Drawing for the job (mm, zero at the part's lowest x, y, z). A direction names the side the tool comes from. Give positions to 0.01 mm unless a question says otherwise; leave off trailing zeros. Order: outer loops, then holes, each group sorted by start corner. A loop starts at its lowest first (then second) coordinate and runs counter-clockwise, first axis right, second up. Notation, with made-up numbers: (89.25, 46.25) - (143.25, 46.25) arc R12 cw to (143.25, 68.25) - close; hole circle Ø9 at (45, 19). An arc over 180 degrees is marked (long way). Use CSV: the item, a comma, the result in double quotes. Start each with the question number.
(1) Band-saw the part on B-B, the plane x = 3.66. Give the cut face in (y, z).
(2) Band-saw the part on D-D, the plane x = 23.66. Give the cut face in (y, z), then the cut area to 3 significant figures.
(3) Band-saw the part on A-A, the plane y = 17. Give the cut face in (x, z), then the cut area to 3 significant figures.
(4) Drop flat-ended pins along their axis: pin 1 Ø6 at (x, y) = (41.5, 30.5) entering from -Z; pin 2 Ø2.5 at (x, z) = (5, 3.5) entering from +Y; pin 3 Ø1.5 at (x, z) = (3, 2) entering from -Y; pin 4 Ø2 at (x, y) = (12.5, 20.5) entering from +Z. Give the stop position or say it passes through.
(5) Pull direction X, two halves, no side cores. Call the marked faces 1, 2, 3 and 4: +X half, -X half, draft (parallel to the pull), parting line (faces both ways), or undercut.
(6) Probe L1, parallel to X at y = 17, z = 1.5; L2, parallel to Y at x = 23.66, z = 3.1; L3, parallel to Y at x = 16.5, z = 3.2. List the from-to ranges inside material, lowest first.
(7) Band-saw the part on C-C, the plane z = 1.6. Give the cut face in (x, y).
(8) Tool access for the marked faces 5, 6 and 7: list every direction of +Z, -Z, +X, -X, +Y, -Y with a clear straight run to the whole face (end or side of a thin tool).
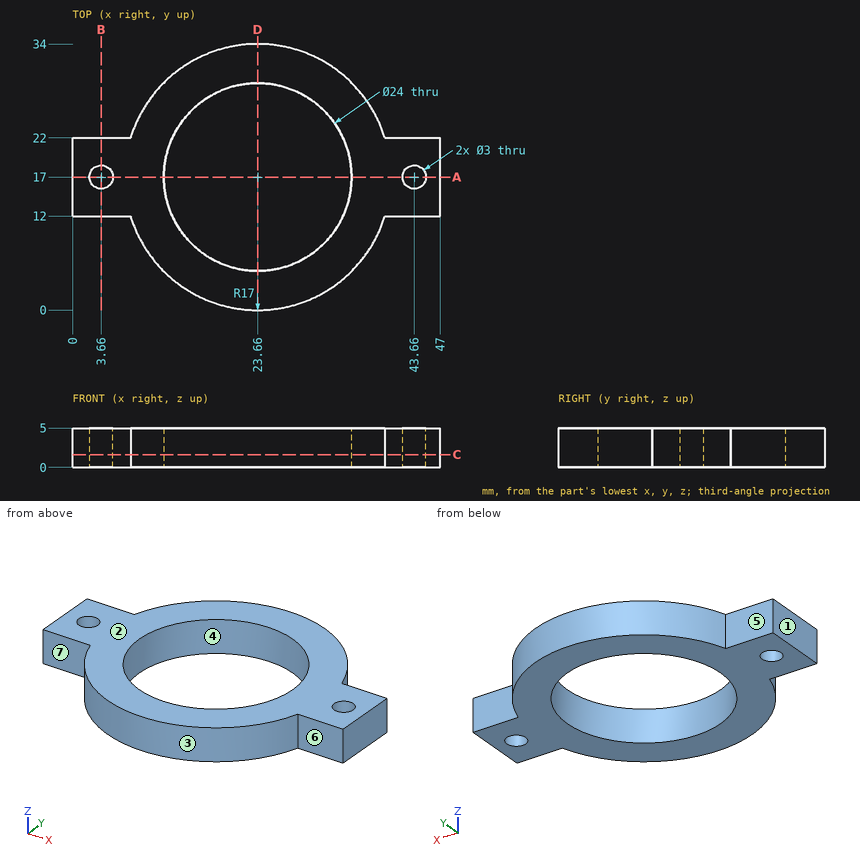
Answer block:
1,outline,"(12, 0) - (15.5, 0) - (15.5, 5) - (12, 5) - close; (18.5, 0) - (22, 0) - (22, 5) - (18.5, 5) - close"
2,outline,"(0, 0) - (5, 0) - (5, 5) - (0, 5) - close; (29, 0) - (34, 0) - (34, 5) - (29, 5) - close"
2,area,"50.0 mm2"
3,outline,"(0, 0) - (2.16, 0) - (2.16, 5) - (0, 5) - close; (5.16, 0) - (11.66, 0) - (11.66, 5) - (5.16, 5) - close; (35.66, 0) - (42.16, 0) - (42.16, 5) - (35.66, 5) - close; (45.16, 0) - (47, 0) - (47, 5) - (45.16, 5) - close"
3,area,"85.0 mm2"
4,pin 1,"passes through"
4,pin 2,"stops at y = 22"
4,pin 3,"stops at y = 12"
4,pin 4,"stops at z = 5"
5,face 1,"-X half"
5,face 2,"draft"
5,face 3,"parting line"
5,face 4,"undercut"
6,L1,"x = 0 to 2.16, 5.16 to 11.66, 35.66 to 42.16, 45.16 to 47"
6,L2,"y = 0 to 5, 29 to 34"
6,L3,"y = 1.58 to 7.37, 26.63 to 32.42"
7,outline,"(0, 12) - (7.41, 12) arc R17 ccw to (39.91, 12) - (47, 12) - (47, 22) - (39.91, 22) arc R17 ccw to (7.41, 22) - (0, 22) - close; hole circle Ø3 at (3.66, 17); hole circle Ø24 at (23.66, 17); hole circle Ø3 at (43.66, 17)"
8,face 5,"+Z, -Z, -X, +Y"
8,face 6,"+Z, -Z, +X, -Y"
8,face 7,"+Z, -Z, -X, -Y"
